Could you check a few things on this drawing? It's one solid part, dimensions in mm from its lowest x, y, z. Give positions to 0.01 mm unless a question says otherwise; leave off trailing zeros. Write each loop counter-clockwise with the first axis right and the second up, starting at its lowest first coordinate (ties: lowest second). Pieces come first, ordered by that corner, then holes. Notation, with made-up numbers: M 81.25,-18.75 L 130.25,-18.75 A19 cw 130.25,0.25 Z; hole C -10,85.5 d10. An arc over 180 degrees is marked long. Answer as CSV lines item,"result". Start each with the question number.
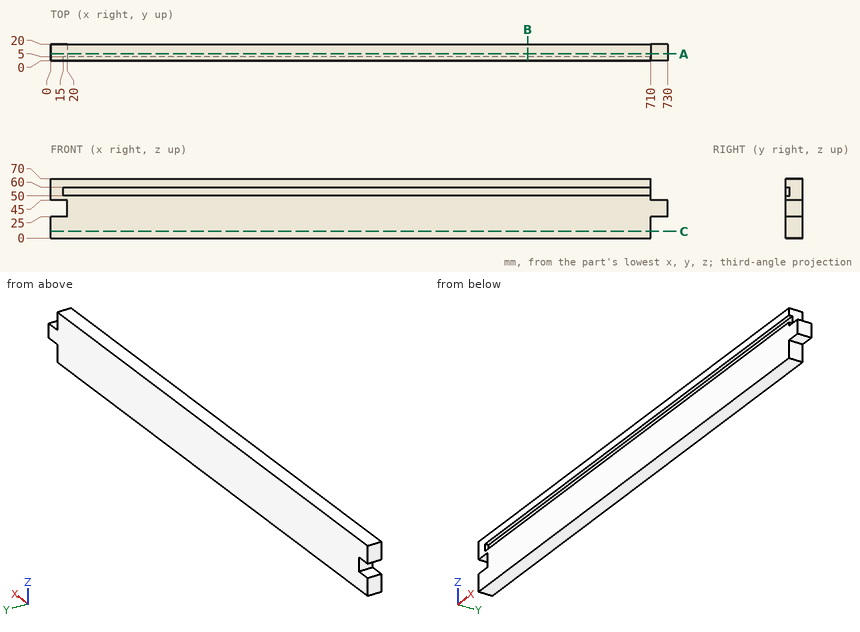
1) I want a section at A-A, the plane y = 8.25. Please give me the cut outline in (x, z), then the cut area to 3 significant figures.
2) I want a section at C-C, the plane z = 8. Please give me the cut outline in (x, y), then the cut area to 3 significant figures.
3) I'm going to push flat-ended pins straight in: P1, Ø3, axis at y = 4, z = 31.5, coming from the -X side; P2, Ø10, axis at x = 716, y = 5.5, coming from the -Z side; P3, Ø10, axis at y = 8, z = 61, coming from the +X side. Where does each tip first touch, or does it pass through?
4) I need wall thicknesses on L1, parallel to Z at x = 131.5, y = 1.5; L2, parallel to X at y = 12.25, z = 39; L3, parallel to Y at x = 54, z = 54.5. Which ranges of each line are inside material? Lowest first, please. Write a range as from..to.
5) I want a section at B-B, the plane x = 564.5. Please give me the cut outline in (y, z).
Values found:
1,outline,"M 0,0 L 710,0 L 710,25 L 730,25 L 730,45 L 710,45 L 710,70 L 0,70 L 0,45 L 20,45 L 20,25 L 0,25 Z"
1,area,"49,700 mm²"
2,outline,"M 0,0 L 710,0 L 710,20 L 0,20 Z"
2,area,"14,200 mm²"
3,P1,"stops at x = 20"
3,P2,"stops at z = 25"
3,P3,"stops at x = 710"
4,L1,"z = 0..50, 60..70"
4,L2,"x = 20..730"
4,L3,"y = 5..20"
5,outline,"M 0,0 L 20,0 L 20,70 L 0,70 L 0,60 L 5,60 L 5,50 L 0,50 Z"
